from build123d import *

# Parameters (mm, degrees)
F0_W     = 10
F0_H     = 60
F1_DEPTH = 10
F3_D     = 4.4
F3_DEPTH = 3.6
F3_TIP   = 1.3218933619
F4_R     = 2


with BuildPart() as f1:
    # F0 (on Front) → F1 (new body)
    with BuildSketch(Plane.XZ):
        Rectangle(F0_W, F0_H)
    extrude(amount=F1_DEPTH)

    # F3
    with Locations(Plane(origin=(0, 0, -30), x_dir=(1, 0, 0), z_dir=(0, 0, -1))):
        with Locations((0, 5.1514371298)):
            Hole(F3_D / 2, depth=F3_DEPTH)
            with Locations((0, 0, -(F3_DEPTH + F3_TIP / 2))):  # 118° drill point
                Cone(0, F3_D / 2, F3_TIP, mode=Mode.SUBTRACT)

    # F4
    f4_edges = [f1.edges().sort_by_distance(p)[0] for p in [
        (5, -5, 30),
        (-5, -5, 30),
        (0, 0, 30),
        (0, -10, 30),
    ]]
    fillet(f4_edges, radius=F4_R)


solid = f1.part
Design review of the part built by this model. Coordinates are the model's own, in mm. A direction names the side the tool comes from. Coordinates: 2 decimals unless noted, no trailing zeros.
Item 1: Clearance check with a flat-ended pin moving along its axis: pin 1 (4 mm diameter, centred on x = -1.5, z = 14, fed in from +Y). State where the tip first meets the part, or that it passes through.
Completed:
pin 1: stops at y = 0
Item 2: Draft analysis for pull direction X (two halves, no side actions). For faces 1 (the cylindrical face through (4.4, -5.07, 29.43)), 2 (the conical face through (-0.083, -4.778, -25.308)), 3 (the flat face through (-5, -5, -1)), 4 (the flat face through (0, -10, -1)), state which applies: pulls with the +X half, pulls with the -X half, needs draft (parallel to the pull), parting line crosses it, or undercut.
Completed:
face 1: pulls with the +X half
face 2: undercut
face 3: pulls with the -X half
face 4: needs draft
Item 3: For faces 5 (the flat face through (-0.1, -2.7, -30)), 6 (the cylindrical face through (-1.18, -7.01, -28.17)), list the 3-axis set-ups (+Z, -Z, +X, -X, +Y, -Y) from which the entire face can be reached by the end or side of a thin tool; tool diameter is ignored.
Completed:
face 5: -Z, +X, -X, +Y, -Y
face 6: -Z
Item 4: Wall thickness on L1, parallel to Y at x = 0, z = -28.2; L2, parallel to Z at x = -1.25, y = -4.25; L3, parallel to Z at x = 3.5, y = -6: over which ranges is each line inside the solid? List them lowest first.
Completed:
L1: y = -10 to -7.35, -2.95 to 0
L2: z = -26 to 30
L3: z = -30 to 29.94
